The listing builds one solid part. Answer for the finished solid, in the listing's coordinates (mm). Face numbers are marked on the shaded views. A direction names the side the tool comes from. Give positions to 0.01 mm unless a question says otherwise; leave off trailing zeros. Write each loop counter-clockwise with the first axis right and the second up, starting at its lowest first coordinate (ties: lowest second). Pieces come first, ordered by that corner, then holes. Notation, with made-up numbers: (77.5, 48) - (124.5, 48) arc R21 ccw to (124.5, 75) - close; hole circle Ø8 at (-39, -31.75). An arc over 180 degrees is marked (long way). One line per item, written item: value. Start each with the question number.
Autodesk Inventor part; units mm, degrees
ref_plane "YZ Plane" through (0, 0, 0) normal (1, 0, 0) x (0, 1, 0)
ref_plane "XZ Plane" through (0, 0, 0) normal (0, 1, 0) x (-1, 0, 0)
ref_plane "XY Plane" through (0, 0, 0) normal (0, 0, 1) x (1, 0, 0)
sketch "スケッチ1" plane through (0, 0, 0) normal (0, 0, 1) x (1, 0, 0)
  line L0 (0, 0) -> (0, 23.3181) construction
  line L1 (-22.6457, 15.5) -> (22.6457, 15.5) construction
  line L2 (-20.3832, 1.5) -> (20.3832, 1.5) construction
  circle A0 centre (0, 15.5) radius 14 construction
  line L3 (-22.6457, 7.5) -> (22.6457, 7.5) construction
  circle A1 centre (-17.5, 15.5) radius 2.1
  circle A2 centre (17.5, 15.5) radius 2.1
  line L4 (-21.5, 20) -> (-21.5, 0)
  line L5 (-21.5, 0) -> (-14.25, 0)
  line L6 (-14.25, 0) -> (-14.25, 20)
  line L7 (21.5, 20) -> (21.5, 0)
  line L8 (21.5, 0) -> (14.25, 0)
  line L9 (14.25, 0) -> (14.25, 20)
  line L10 (-14.25, 20) -> (-21.5, 20)
  line L11 (14.25, 20) -> (21.5, 20)
  line L12 (21.5, 1.5) -> (-21.5, 1.5)
  line L13 (-21.5, 1.5) -> (-21.5, 0)
  line L14 (-21.5, 0) -> (21.5, 0)
  line L15 (21.5, 0) -> (21.5, 1.5)
  point P0 (0, 1.5)
  point P1 (0, 7.5)
  point P2 (14.25, 1.5)
  point P3 (-14.25, 1.5)
  dimension "d0" = 28
  dimension "d1" = 1.5
  dimension "d2" = 8
  dimension "d3" = 4.2
  dimension "d4" = 35
  dimension "d6" = 20
  dimension "d29" = 3.25
  dimension "d30" = 3.25
  dimension "d31" = 4
  dimension "d32" = 4
extrude "前" add sketch "スケッチ1" along normal blind 2
extrude "底" add sketch "スケッチ1" against normal blind 15 contours L12 L6 L5 L4 | L12 L9 L14 L6 | L12 L7 L8 L9
sketch "スケッチ5" plane through (-14.25, 1.5, 2) normal (0, 1, 0) x (1, 0, 0)
  line L0 (14.25, -6.214) -> (14.25, 25.3742) construction
  line L1 (28.5, 0) -> (0, 0) construction
  point P0 (14.25, 2)
  point P1 (-3.25, 14)
  point P2 (31.75, 14)
  dimension "d33" = 35
  dimension "d34" = 14
hole "穴2" at (-17.5, 1.5, -12) at (17.5, 1.5, -12) direction (0, -1, 0) diameter 3.2 end through all
sketch "スケッチ6" plane through (21.5, 1.5, 0) normal (1, 0, 0) x (0, 0, -1)
  line L0 (2, 18.5) -> (-2, 18.5)
  line L1 (-2, 18.5) -> (-2, 0)
  line L2 (-2, 18.5) -> (-2, -1.5)
  line L3 (-2, -1.5) -> (8, -1.5)
  line L4 (8, -1.5) -> (8, 0)
  line L5 (8, 0) -> (2, 18.5)
  point P0 (0, -1.5)
  point P1 (15, 0)
  dimension "d42" = 4
  dimension "d43" = 10
extrude "押し出し5" add sketch "スケッチ6" along normal blind 0.8
mirror "ミラー3" about plane through (0, 0, 0) normal (1, 0, 0) of "押し出し5"
equation "\"d30\" = d29"
equation "\"d32\" = d31"
properties part number "28BYJ-48_Braket2"
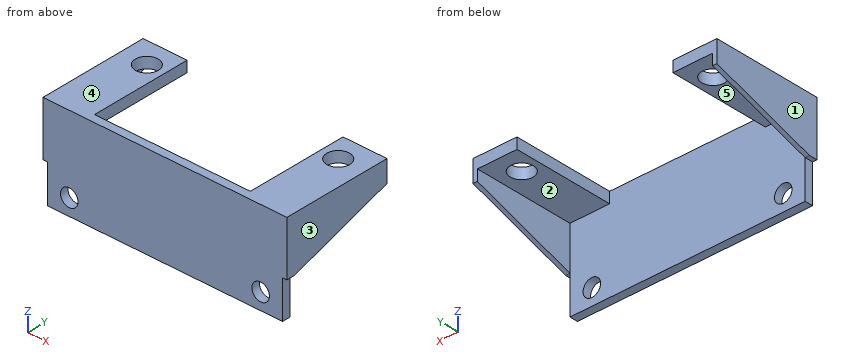
Item 1: Straight lines are drawn through the part: line 1 along X through (y, z) = (0.85, -12); line 2 along X through (y, z) = (14.5, -3.5); line 3 along Z through (x, y) = (17.5, 1.1). For each, find the intervals that lie inside material, in ascending order.
Item 2: Find section A-A on z = -12. Determine the outline of the cut face in (x, y), plus the area to 3 significant figures.
Item 3: The mould has two halves that part along X. Classify the marked faces 1, 2 and 3: +X half, -X half, draft (parallel to the pull), parting line (faces both ways), or undercut.
Item 4: Find section D-D on y = 15.5. Determine the outline of the cut face in (x, z), plus the area to 3 significant figures.
Item 5: For the marked faces 4 and 5, determine the directions among +Z, -Z, +X, -X, +Y, -Y from which every point of the face is accessible in a straight line to the end or side of a thin tool.
Item 6: Find section C-C on y = 2. Determine the outline of the cut face in (x, z).
Item 7: Find section B-B on x = -17.5. Determine the outline of the cut face in (y, z), plus the area to 3 significant figures.
Item 8: Each of these flat-tipped pins is pushed along its axis until it touches: pin 1 Ø5 at (x, z) = (-8, -1.5) entering from +Y; pin 2 Ø8 at (x, y) = (-17, 9) entering from -Z; pin 3 Ø4 at (x, y) = (-17.5, 15.5) entering from -Z; pin 4 Ø1.6 at (y, z) = (0.5, -12) entering from +X. Where does it stop, or does it pass through?
Values:
1. line 1: -21.5 to -19.1, -15.9 to 15.9, 19.1 to 21.5
1. line 2: -22.3 to -21.5, 21.5 to 22.3
1. line 3: -15 to -13.6, -10.4 to 2
2. outline: (-21.5, 0) - (-19.1, 0) - (-19.1, 1.5) - (-21.5, 1.5) - close; (-15.9, 0) - (15.9, 0) - (15.9, 1.5) - (-15.9, 1.5) - close; (19.1, 0) - (21.5, 0) - (21.5, 1.5) - (19.1, 1.5) - close
2. area: 54.9 mm^2
3. face 1: -X half
3. face 2: undercut
3. face 3: +X half
4. outline: (-22.3, -3.46) - (-21.5, -3.46) - (-21.5, 0) - (-19.6, 0) - (-19.6, 2) - (-22.3, 2) - close; (-15.4, 0) - (-14.25, 0) - (-14.25, 2) - (-15.4, 2) - close; (14.25, 0) - (15.4, 0) - (15.4, 2) - (14.25, 2) - close; (19.6, 0) - (21.5, 0) - (21.5, -3.46) - (22.3, -3.46) - (22.3, 2) - (19.6, 2) - close
4. area: 20.9 mm^2
5. face 4: +Z, +X, -X, +Y, -Y
5. face 5: -Z, +Y
6. outline: (-22.3, -7.84) - (-21.5, -7.84) - (-21.5, 0) - (-14.25, 0) - (-14.25, 2) - (-22.3, 2) - close; (14.25, 0) - (21.5, 0) - (21.5, -7.84) - (22.3, -7.84) - (22.3, 2) - (14.25, 2) - close
7. outline: (0, -15) - (1.5, -15) - (1.5, -13.6) - (0, -13.6) - close; (0, -10.4) - (1.5, -10.4) - (1.5, 0) - (13.4, 0) - (13.4, 2) - (0, 2) - close; (17.6, 0) - (20, 0) - (20, 2) - (17.6, 2) - close
7. area: 49.3 mm^2
8. pin 1: y = 1.5
8. pin 2: z = 0
8. pin 3: through
8. pin 4: x = 21.5
